```python
from build123d import *

# Parameters (mm, degrees)
SKETCH_1_R      = 2.5
EXTRUDE_1_DEPTH = 300
FILLET_1_R      = 1.5


with BuildPart() as part:
    # 草图1 → 凸台-拉伸1 (new body)
    with BuildSketch(Plane(origin=(0, 0, 0), x_dir=(1, 0, 0), z_dir=(0, 1, 0))):
        Polygon((10, 10), (3.65, 10), (3.65, 9.303257497), (3.1, 9.303257497), (3.1, 8.2), (5.6, 8.2), (5.6, 6.660660172), (2.839339828, 3.9), (-2.839339828, 3.9), (-5.6, 6.660660172), (-5.6, 8.2), (-3.1, 8.2), (-3.1, 9.303257497), (-3.65, 9.303257497), (-3.65, 10), (-10, 10), (-10, 3.65), (-9.303257497, 3.65), (-9.303257497, 3.1), (-8.2, 3.1), (-8.2, 5.6), (-6.660660172, 5.6), (-3.9, 2.839339828), (-3.9, -2.839339828), (-6.660660172, -5.6), (-8.2, -5.6), (-8.2, -3.1), (-9.303257497, -3.1), (-9.303257497, -3.65), (-10, -3.65), (-10, -10), (-3.65, -10), (-3.65, -9.303257497), (-3.1, -9.303257497), (-3.1, -8.2), (-5.6, -8.2), (-5.6, -6.660660172), (-2.839339828, -3.9), (2.839339828, -3.9), (5.6, -6.660660172), (5.6, -8.2), (3.1, -8.2), (3.1, -9.303257497), (3.65, -9.303257497), (3.65, -10), (10, -10), (10, -3.65), (9.303257497, -3.65), (9.303257497, -3.1), (8.2, -3.1), (8.2, -5.6), (6.660660172, -5.6), (3.9, -2.839339828), (3.9, 2.839339828), (6.660660172, 5.6), (8.2, 5.6), (8.2, 3.1), (9.303257497, 3.1), (9.303257497, 3.65), (10, 3.65), align=None)
        with Locations(Location((0, 0, 0), (0, 0, 270))):
            Circle(SKETCH_1_R, mode=Mode.SUBTRACT)
    extrude(amount=EXTRUDE_1_DEPTH)

    # 圆角1
    fillet_1_edges = [part.edges().sort_by_distance(p)[0] for p in [
        (10, 150, 10),
        (-10, 150, 10),
        (-10, 150, -10),
        (10, 150, -10),
    ]]
    fillet(fillet_1_edges, radius=FILLET_1_R)


solid = part.part
```
Can you work these out from the model? Positions are in its coordinate system, mm. A direction names the side the tool comes from. Give positions to 0.01 mm unless a question says otherwise; leave off trailing zeros. Loops run counter-clockwise (first coordinate to the right, second up) from the corner with the lowest first, then second, coordinate; pieces in that order, holes last. Notation, with made-up numbers: M -28,-29 L 11,-29 A24 ccw 11,-14 Z; hole C 53,27 d6. An arc over 180 degrees is marked long. Use one line per item in the form item = value. Start each with the question number.
(1) I want a section at A-A, the plane x = 0. Write out the boundary of the cut face in (y, z), and give its area (3 significant figures).
(2) Thinking about a two-plate mould opening in X: for faces 1 (the flat face through (10, 148, 6)), 2 (the flat face through (0, 148, -3.9)), 3 (the flat face through (-10, 148, 6)), which applies, released by +X, released by -X, zero draft, split by the parting line, or undercut?
(3) I'm going to push flat-ended pins straight in: P1, Ø8, axis at y = 139.5, z = 2.5, coming from the +X side; P2, Ø0.8, axis at y = 155, z = -10, coming from the +X side; P3, Ø4, axis at x = 0.5, y = 259.5, coming from the +Z side; P4, Ø0.6, axis at x = 9.5, y = 189.5, coming from the +Z side. Where does each tip first touch, or does it pass through?
(4) Please list where these lines run through material, in increasing order: line 1 (Z direction, x = 8, y = 203); line 2 (Z direction, x = -5, y = 51); line 3 (X direction, y = 262, z = 3.5).
(5) On a 3-axis mill with a long thin cutter (end or side, diameter ignored), from which of +Z, -Z, +X, -X, +Y, -Y can I reach the whole of each face in a straight line? I mean faces 4 (the flat face through (-3.9, 148, 0)), 5 (the flat face through (0, 148, 3.9)), 6 (the flat face through (3.9, 148, 0)). Say none if no direction works.
(6) I want a section at B-B, the plane z = 0. Write out the boundary of the cut face in (x, y).
Worked out:
q1.outline = M 0,-3.9 L 300,-3.9 L 300,-2.5 L 0,-2.5 Z; M 0,2.5 L 300,2.5 L 300,3.9 L 0,3.9 Z
q1.area = 840 mm²
q2.face_1 = released by +X
q2.face_2 = undercut
q2.face_3 = released by -X
q3.P1 = 10
q3.P2 = 9.52
q3.P3 = 3.9
q3.P4 = 9.83
q4.line_1 = -10 to -5.6, 5.6 to 10
q4.line_2 = -10 to -8.2, -6.06 to -3.94, 3.94 to 6.06, 8.2 to 10
q4.line_3 = -9.3 to -8.2, -4.56 to 4.56, 8.2 to 9.3
q5.face_4 = -X, +Y, -Y
q5.face_5 = +Z, +Y, -Y
q5.face_6 = +X, +Y, -Y
q6.outline = M -3.9,0 L -2.5,0 L -2.5,300 L -3.9,300 Z; M 2.5,0 L 3.9,0 L 3.9,300 L 2.5,300 Z
